CAD build for the part. Positions are in the model's coordinates, mm. A direction names the side the tool comes from. Round coordinates to 2 decimals unless told otherwise and drop trailing zeros. Loops run counter-clockwise (first coordinate to the right, second up) from the corner with the lowest first, then second, coordinate; pieces in that order, holes last.
```python
from build123d import *

# Parameters (mm, degrees)
EXTRUDE_1_DEPTH     = 20
EXTRUDE_2_DEPTH     = 2.6
SKETCH_3_W          = 6
SKETCH_3_H          = 2
EXTRUDE_3_DEPTH     = 1.5
SKETCH_4_R          = 3
CUT_EXTRUDE_1_DEPTH = 4


with BuildPart() as part:
    # 草图1 → 凸台-拉伸1 (new body)
    with BuildSketch(Plane.XY):
        Polygon((0, 0), (0, 28), (4, 28), (4, 4), (28, 4), (28, 0), align=None)
    extrude(amount=EXTRUDE_1_DEPTH)

    # 草图2 → 凸台-拉伸2 (add)
    with BuildSketch(Plane.XY.offset(20)):
        Polygon((4, 28), (6, 28), (6, 23), (23, 6), (28, 6), (28, 4), (4, 4), align=None)
    extrude_2 = extrude(amount=-EXTRUDE_2_DEPTH)

    # 镜向1: 凸台-拉伸2 across plane
    add(extrude_2.mirror(Plane(origin=(0, 0, 10), x_dir=(1, 0, 0), z_dir=(0, 0, -1))))

    # 草图3 → 凸台-拉伸3 (add)
    with BuildSketch(Plane.ZY):
        with Locations((10, 25)):
            Rectangle(SKETCH_3_W, SKETCH_3_H)
        with Locations((10, 3)):
            Rectangle(SKETCH_3_W, SKETCH_3_H)
    extrude_3 = extrude(amount=EXTRUDE_3_DEPTH)

    # 镜向2: 凸台-拉伸3 across plane
    add(extrude_3.mirror(Plane(origin=(0, 0, 0), x_dir=(0, 0, 1), z_dir=(-0.707106781, 0.707106781, 0))))

    # 草图4 → 切除-拉伸1 (cut)
    with BuildSketch(Plane.ZY):
        with Locations((10, 17)):
            Circle(SKETCH_4_R)
    cut_extrude_1 = extrude(amount=-CUT_EXTRUDE_1_DEPTH, mode=Mode.SUBTRACT)

    # 镜向3: 切除-拉伸1 across plane
    add(cut_extrude_1.mirror(Plane(origin=(0, 0, 0), x_dir=(0, 0, 1), z_dir=(-0.707106781, 0.707106781, 0))), mode=Mode.SUBTRACT)


solid = part.part
```
Item 1: Cut at A-A, the plane z = 10. State how many separate pieces and enclosed holes the cut face has, plus the area to 3 significant figures.
Answers follow:
separate pieces: 3
enclosed holes: 0
area: 172 mm2
Item 2: 3-axis set-ups, long thin cutter, end or side, ignore diameter. For faces 1 (the flat face through (11, 11, 17.4)), 2 (the flat face through (24, -1, 10)), 3 (the flat face through (-1, 25, 13)): which of +Z, -Z, +X, -X, +Y, -Y reach the whole face in a straight line?
Answers follow:
face 1: +X, +Y
face 2: +Z, -Z, -Y
face 3: +Z, -X, +Y, -Y
Item 3: Flat gauge pins, fed straight in: P1, Ø1.3, axis at x = 25, z = 1, coming from the +Y side; P2, Ø3, axis at x = 6, y = 17, coming from the -Z side; P3, Ø12, axis at x = 14, z = 13, coming from the +Y side; P4, Ø3, axis at y = 7.5, z = 14, coming from the -X side. Where does each tip first touch, or does it go through?
Answers follow:
P1: stops at y = 6
P2: stops at z = 0
P3: stops at y = 19.08
P4: stops at x = 0
Item 4: Cut at D-D, the plane x = 1. Give the cut face in (y, z), plus the area to 3 significant figures.
Answers follow:
outline: (0, 0) - (28, 0) - (28, 20) - (0, 20) - close; hole circle Ø6 at (17, 10)
area: 532 mm2
Item 5: Cut at B-B, the plane y = 17. Give the cut face in (x, z).
Answers follow:
outline: (0, 0) - (12, 0) - (12, 2.6) - (4, 2.6) - (4, 7) - (0, 7) - close; (0, 13) - (4, 13) - (4, 17.4) - (12, 17.4) - (12, 20) - (0, 20) - close
Item 6: Two-plate mould, pull along Y, no slides. Class faces 4 (the flat face through (2, 28, 10)), 5 (the cylindrical face through (1.972, 14.338, 11.384)), 6 (the flat face through (3, -1, 13)): released by +Y, released by -Y, zero draft, split by the parting line, or undercut.
Answers follow:
face 4: released by +Y
face 5: undercut
face 6: zero draft
Item 7: Probe line 1 (X direction, y = 2.4, z = 10); line 2 (X direction, y = 1.3, z = 10). List the from-to ranges inside material, lowest first.
Answers follow:
line 1: x = -1.5 to 14, 20 to 28
line 2: x = 0 to 14, 20 to 28
